Model file for the job. Use its own axes, mm. A direction names the side the tool comes from. Round coordinates to 2 decimals unless told otherwise and drop trailing zeros. Put each result on its own line as item: value. Start each with the question number.
Item 1: Mould opens along X. For faces 1 (the face through (-304.8, 25, 2)), 2 (the face through (-142.956, 25.353, -1.24)), 3 (the face through (-4, 25, -152.4)), 4 (the face through (301.18, 25.35, -148.58)) say: pulls with the +X half, pulls with the -X half, needs draft (parallel to the pull), parting line crosses it, or undercut.
Item 2: Which spindle directions (+Z, -Z, +X, -X, +Y, -Y) get a long thin tool onto all of the face, cutting with end or side? Do faces 5 (the face through (204.4, 8.7, 36.7)), 6 (the face through (-4, 50.006, -2)). Say none if no direction does.
Item 3: Pin check, flat tip, straight feed: pin 1 Ø11.5 at (x, z) = (222.25, 0) entering from -Y. Stop position of the tip, or through.
Item 4: Probe probe 1 along Z at (x, y) = (-50.8, 31); probe 2 along Z at (x, y) = (-273.05, 4); probe 3 along Z at (x, y) = (272.5, 15). List the from-to ranges inside material, lowest first.
```python
from build123d import *

# Parameters (mm, degrees)
SKETCH1_W                                         = 609.6
SKETCH1_H                                         = 304.8
EXTRUDE1_DEPTH                                    = 50.00625
FILLET1_R                                         = 12.7
SKETCH2_R                                         = 9.525
CUT_EXTRUDE1_DEPTH                                = 345.426225829
CBORE_FOR_5_16_SOCKET_HEAD_CAP_SCREW1_D           = 8.72998
CBORE_FOR_5_16_SOCKET_HEAD_CAP_SCREW1_CBORE_D     = 13.49502
CBORE_FOR_5_16_SOCKET_HEAD_CAP_SCREW1_CBORE_DEPTH = 8.6995
F_3_8_16_TAPPED_HOLE1_D                           = 7.9375
F_3_8_16_TAPPED_HOLE1_DEPTH                       = 26.9875
F_3_8_16_TAPPED_HOLE1_TIP                         = 2.384665582


with BuildPart() as part:
    # Sketch1 → Extrude1 (new body)
    with BuildSketch(Plane(origin=(0, 0, 0), x_dir=(1, 0, 0), z_dir=(0, 1, 0))):
        Rectangle(SKETCH1_W, SKETCH1_H)
    extrude(amount=EXTRUDE1_DEPTH)

    # Fillet1
    fillet1_edges = [part.edges().sort_by_distance(p)[0] for p in [
        (-304.8, 25.003125, -152.4),
        (304.8, 25.003125, -152.4),
        (304.8, 25.003125, 152.4),
        (-304.8, 25.003125, 152.4),
    ]]
    fillet(fillet1_edges, radius=FILLET1_R)

    # Sketch2 → Cut-Extrude1 (cut, through all)
    with BuildSketch(Plane(origin=(0, 50.00625, 0), x_dir=(-1, 0, 0), z_dir=(0, 1, 0))):
        with Locations(Location((152.4, 0, 0), (0, 0, 90))):
            Circle(SKETCH2_R)
        with Locations(Location((-152.4, 0, 0), (0, 0, 90))):
            Circle(SKETCH2_R)
    extrude(amount=-CUT_EXTRUDE1_DEPTH, mode=Mode.SUBTRACT)

    # CBORE for 5/16 Socket Head Cap Screw1 (through all)
    with Locations(Plane.XZ):
        with Locations((-200.025, 38.1), (-200.025, -38.1), (200.025, -38.1), (200.025, 38.1), (-222.25, 0), (-273.05, 0), (222.25, 0), (273.05, 0)):
            CounterBoreHole(CBORE_FOR_5_16_SOCKET_HEAD_CAP_SCREW1_D / 2, CBORE_FOR_5_16_SOCKET_HEAD_CAP_SCREW1_CBORE_D / 2, CBORE_FOR_5_16_SOCKET_HEAD_CAP_SCREW1_CBORE_DEPTH)

    # 3/8-16 Tapped Hole1
    with Locations(Plane(origin=(0, 50.00625, 0), x_dir=(-1, 0, 0), z_dir=(0, 1, 0))):
        with Locations((50.8, 50.8), (50.8, -50.8), (-50.8, -50.8), (-50.8, 50.8), (0, 0)):
            Hole(F_3_8_16_TAPPED_HOLE1_D / 2, depth=F_3_8_16_TAPPED_HOLE1_DEPTH)
            with Locations((0, 0, -(F_3_8_16_TAPPED_HOLE1_DEPTH + F_3_8_16_TAPPED_HOLE1_TIP / 2))):  # 118° drill point
                Cone(0, F_3_8_16_TAPPED_HOLE1_D / 2, F_3_8_16_TAPPED_HOLE1_TIP, mode=Mode.SUBTRACT)


solid = part.part
```
Results found:
1. face 1: pulls with the -X half
1. face 2: undercut
1. face 3: needs draft
1. face 4: pulls with the +X half
2. face 5: -Y
2. face 6: +Z, -Z, +X, -X, +Y
3. pin 1: stops at y = 8.7
4. probe 1: z = -152.4 to -54.77, -46.83 to 46.83, 54.77 to 152.4
4. probe 2: z = -152.4 to -6.75, 6.75 to 152.4
4. probe 3: z = -152.4 to -4.33, 4.33 to 152.4
